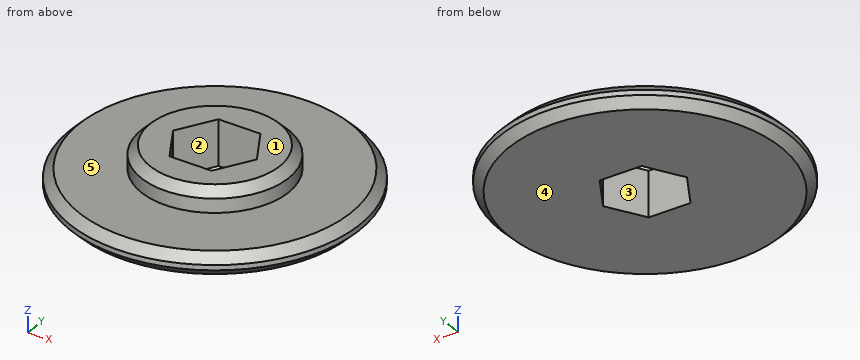
Autodesk Inventor part; units mm, degrees
ref_plane "YZ Plane" through (0, 0, 0) normal (1, 0, 0) x (0, 1, 0)
ref_plane "XZ Plane" through (0, 0, 0) normal (0, 1, 0) x (-1, 0, 0)
ref_plane "XY Plane" through (0, 0, 0) normal (0, 0, 1) x (1, 0, 0)
sketch "Sketch1" plane through (0, 0, 0) normal (0, 0, 1) x (1, 0, 0)
  circle A0 centre (0, 0) radius 24.9555
  line L0 (3.7176, 6.32) -> (7.3321, -0.0596)
  line L1 (7.3321, -0.0596) -> (3.6145, -6.3796)
  line L2 (3.6145, -6.3796) -> (-3.7176, -6.32)
  line L3 (-3.7176, -6.32) -> (-7.3321, 0.0596)
  line L4 (-7.3321, 0.0596) -> (-3.6145, 6.3796)
  line L5 (-3.6145, 6.3796) -> (3.7176, 6.32)
  dimension "d0" = 49.911
  dimension "d14" = 6.35
extrude "Extrusion3" add sketch "Sketch1" along normal blind 3.937
chamfer "Chamfer3" distance 1.524 angle 45 1 edges at (-24.9555, 0, 3.937)
chamfer "Chamfer4" distance 1.524 angle 45 1 edges at (-24.9555, 0, 0)
sketch "Sketch4" plane through (0, 0, 3.937) normal (0, 0, 1) x (1, 0, 0)
  circle A0 centre (0, 0) radius 23.4315
  line L0 (3.7176, 6.32) -> (7.3321, -0.0596)
  line L1 (7.3321, -0.0596) -> (3.6145, -6.3796)
  line L2 (3.6145, -6.3796) -> (-3.7176, -6.32)
  line L3 (-3.7176, -6.32) -> (-7.3321, 0.0596)
  line L4 (-7.3321, 0.0596) -> (-3.6145, 6.3796)
  line L5 (-3.6145, 6.3796) -> (3.7176, 6.32)
  circle A1 centre (0, 0) radius 12.7
  dimension "d23" = 25.4
extrude "Extrusion4" add sketch "Sketch4" along normal blind 3.937 contours A1
chamfer "Chamfer5" distance 1.524 angle 45 1 edges at (-12.7, 0, 7.874)
properties part number "Sprocket Large"
Can you work these out from the model? Positions are in its coordinate system, mm. Face numbers are marked on the shaded views. A direction names the side the tool comes from. Give positions to 0.01 mm unless a question says otherwise; leave off trailing zeros. Order: outer loops, then holes, each group sorted by start corner. A loop starts at its lowest first (then second) coordinate and runs counter-clockwise, first axis right, second up. Notation, with made-up numbers: (44.5, 14) - (60.5, 14) arc R25 ccw to (60.5, 30) - close; hole circle Ø11 at (81.25, -20). An arc over 180 degrees is marked (long way). Use a Markdown table: item, result. Add a question column.
Q1. I'm going to push flat-ended pins straight in: pin 1 (12 mm diameter, centred on x = 18, y = -7.5, fed in from +Z); pin 2 (2 mm diameter, centred on x = -11.5, z = 3.5, fed in from -Y); pin 3 (4 mm diameter, centred on x = -10.5, z = 5, fed in from +Y); pin 4 (4 mm diameter, centred on x = -15, z = 6.5, fed in from -Y). Where does each tip first touch, or does it pass through?
Q2. If we mould it in two halves opening along Y, with no side actions, what happens to the marked faces 1 and 2? For each: released by +Y, released by -Y, zero draft, split by the parting line, or undercut.
Q3. If we section it at C-C on z = 3: Write out the boundary of the cut face in (x, y), plus the area to 3 significant figures.
Q4. On a 3-axis mill with a long thin cutter (end or side, diameter ignored), from which of +Z, -Z, +X, -X, +Y, -Y can I reach the whole of each face in a straight line? I mean the marked faces 3, 4 and 5. Say none if no direction works.
Q5. Please list where these lines run through material, in increasing order: line 1 along Z through (x, y) = (-19, -11.5); line 2 along Y through (x, z) = (-3, 6); line 3 along Z through (x, y) = (22.5, 7).
Q6. If we section it at B-B on x = 0: Write out the boundary of the cut face in (y, z).
Q7. If we section it at A-A on z = 7: Write out the boundary of the cut face in (x, y).
Answers follow:
| question | item | result |
|---|---|---|
| 1 | pin 1 | stops at z = 3.94 |
| 1 | pin 2 | stops at y = -22.16 |
| 1 | pin 3 | stops at y = 22.17 |
| 1 | pin 4 | passes through |
| 2 | face 1 | zero draft |
| 2 | face 2 | undercut |
| 3 | outline | circle Ø48.74 at (0, 0); hole (-7.33, 0.06) - (-3.72, -6.32) - (3.61, -6.38) - (7.33, -0.06) - (3.72, 6.32) - (-3.61, 6.38) - close |
| 3 | area | 1,730 mm^2 |
| 4 | face 3 | +Z, -Z |
| 4 | face 4 | -Z, +X, -X, +Y, -Y |
| 4 | face 5 | +Z |
| 5 | line 1 | z = 0 to 3.94 |
| 5 | line 2 | y = -12.34 to -6.33, 6.37 to 12.34 |
| 5 | line 3 | z = 0.13 to 3.8 |
| 6 | outline | (-24.96, 1.52) - (-23.43, 0) - (-6.35, 0) - (-6.35, 7.87) - (-11.18, 7.87) - (-12.7, 6.35) - (-12.7, 3.94) - (-23.43, 3.94) - (-24.96, 2.41) - close; (6.35, 0) - (23.43, 0) - (24.96, 1.52) - (24.96, 2.41) - (23.43, 3.94) - (12.7, 3.94) - (12.7, 6.35) - (11.18, 7.87) - (6.35, 7.87) - close |
| 7 | outline | circle Ø24.1 at (0, 0); hole (-7.33, 0.06) - (-3.72, -6.32) - (3.61, -6.38) - (7.33, -0.06) - (3.72, 6.32) - (-3.61, 6.38) - close |
